```python
from build123d import *

# Parameters (mm, degrees)
SKETCH_1_R      = 15
SKETCH_1_R_2    = 13.5
EXTRUDE_1_DEPTH = 25
SKETCH_2_R      = 21.5
SKETCH_2_R_2    = 13.5
SKETCH_2_R_3    = 2
EXTRUDE_3_DEPTH = 4
FILLET_2_R      = 1


with BuildPart() as part:
    # 草图1 → 凸台-拉伸1 (new body)
    with BuildSketch(Plane.XY):
        Circle(SKETCH_1_R)
        Circle(SKETCH_1_R_2, mode=Mode.SUBTRACT)
    extrude(amount=EXTRUDE_1_DEPTH)

    # 草图2 → 凸台-拉伸3 (add)
    with BuildSketch(Plane.XY.offset(25)):
        Circle(SKETCH_2_R)
        Circle(SKETCH_2_R_2, mode=Mode.SUBTRACT)
        with Locations((0, 18.25)):
            Circle(SKETCH_2_R_3, mode=Mode.SUBTRACT)
        with Locations((18.25, 0)):
            Circle(SKETCH_2_R_3, mode=Mode.SUBTRACT)
        with Locations((0, -18.25)):
            Circle(SKETCH_2_R_3, mode=Mode.SUBTRACT)
        with Locations((-18.25, 0)):
            Circle(SKETCH_2_R_3, mode=Mode.SUBTRACT)
    extrude(amount=EXTRUDE_3_DEPTH)

    # 圆角2
    fillet_2_edges = [part.edges().sort_by_distance(p)[0] for p in [
        (-15, 0, 25),
    ]]
    fillet(fillet_2_edges, radius=FILLET_2_R)


solid = part.part
```
Work out the finished part from the listing and answer in its coordinate system (mm). A direction names the side the tool comes from. Round coordinates to 2 decimals unless told otherwise and drop trailing zeros. Loops run counter-clockwise (first coordinate to the right, second up) from the corner with the lowest first, then second, coordinate; pieces in that order, holes last.
(1) The part is cut by section A-A, the plane y = 0. Give the vertices of the cut face in (x, z), and give its area (3 significant figures).
Computed values:
outline: (-21.5, 25) - (-20.25, 25) - (-20.25, 29) - (-21.5, 29) - close; (-16.25, 25) - (-16, 25) arc R1 cw to (-15, 24) - (-15, 0) - (-13.5, 0) - (-13.5, 29) - (-16.25, 29) - close; (13.5, 0) - (15, 0) - (15, 24) arc R1 cw to (16, 25) - (16.25, 25) - (16.25, 29) - (13.5, 29) - close; (20.25, 25) - (21.5, 25) - (21.5, 29) - (20.25, 29) - close
area: 107 mm2
(2) For faces 4 (the cylindrical face through (16.663, -1.217, 26.972)), 5 (the flat face through (7.9, 14.4, 25)), determine the directions among +Z, -Z, +X, -X, +Y, -Y from which every point of the face is accessible in a straight line to the end or side of a thin tool.
Computed values:
face 4: +Z, -Z
face 5: -Z
(3) The part is cut by section D-D, the plane z = 27.25. Give the vertices of the cut face in (x, y).
Computed values:
outline: circle Ø43 at (0, 0); hole circle Ø4 at (-18.25, 0); hole circle Ø27 at (0, 0); hole circle Ø4 at (0, -18.25); hole circle Ø4 at (0, 18.25); hole circle Ø4 at (18.25, 0)
(4) Each of these flat-tipped pins is pushed along its axis until it touches: P1, Ø4, axis at y = -13, z = 20.5, coming from the -X side; P2, Ø10, axis at x = 3, z = 16.5, coming from the +Y side; P3, Ø3.5, axis at x = -18.25, y = 0, coming from the +Z side; P4, Ø10, axis at x = 7.5, y = 4.5, coming from the -Z side. Where does it stop, or does it pass through?
Computed values:
P1: stops at x = -10.2
P2: stops at y = 15
P3: passes through
P4: stops at z = 0
(5) The mould has two halves that part along X. Classify faces 1 (the flat face through (0, -14, 29)), 2 (the cylindrical face through (-0.26, -16.267, 26.972)), 3 (the cylindrical face through (-14.985, 0.66, 11.832)): pulls with the +X half, pulls with the -X half, needs draft (parallel to the pull), parting line crosses it, or undercut.
Computed values:
face 1: needs draft
face 2: undercut
face 3: parting line crosses it
(6) The part is cut by section B-B, the plane x = 19.5. Give the vertices of the cut face in (y, z).
Computed values:
outline: (-9.06, 25) - (-1.56, 25) - (-1.56, 29) - (-9.06, 29) - close; (1.56, 25) - (9.06, 25) - (9.06, 29) - (1.56, 29) - close
(7) Find the intervals of material crossed by L1, parallel to Y at x = 0, z = 6.5; L2, parallel to Z at x = 15, y = 6; L3, parallel to Y at x = -4, z = 17, in increasing order.
Computed values:
L1: y = -15 to -13.5, 13.5 to 15
L2: z = 25 to 29
L3: y = -14.46 to -12.89, 12.89 to 14.46
